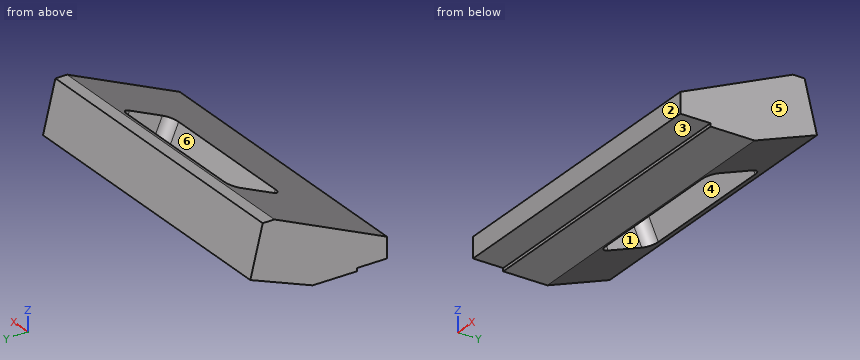
```python
from build123d import *

# Parameters (mm, degrees)
F1_DEPTH = 300
F3_DEPTH = 106


with BuildPart() as f1:
    # F0 (on Right) → F1 (new body)
    with BuildSketch(Plane.YZ):
        Polygon((0, 0), (0, -20), (29.5, -20), (29.5, -23), (72.5, -23), (133.294737, 0), (121.198642, 48.514786), (109.755708, 48.514786), align=None)
    extrude(amount=F1_DEPTH)

    # F2 (on face) → F3 (cut)
    with BuildSketch(Plane(origin=(0, 0, 0), x_dir=(1, 0, 0), z_dir=(0, -0.40429, 0.914631))):
        with BuildLine():
            Line((220, 115), (80, 115))
            ThreePointArc((80, 115), (72.928932, 112.071068), (70, 105))
            Line((70, 105), (70, 70))
            ThreePointArc((70, 70), (72.928932, 62.928932), (80, 60))
            Line((80, 60), (220, 60))
            ThreePointArc((220, 60), (227.071068, 62.928932), (230, 70))
            Line((230, 70), (230, 105))
            ThreePointArc((230, 105), (227.071068, 112.071068), (220, 115))
        make_face()
    extrude(amount=-F3_DEPTH, mode=Mode.SUBTRACT)


solid = f1.part
```
For this review, take the finished solid that the model builds, in its own axes (mm). Face numbers are marked on the shaded views. A direction names the side the tool comes from. Coordinates: 2 decimals unless noted, no trailing zeros. Write each loop counter-clockwise with the first axis right and the second up, starting at its lowest first coordinate (ties: lowest second). Pieces come first, ordered by that corner, then holes. Notation, with made-up numbers: (42.25, -23) - (69.25, -23) arc R14 cw to (69.25, -10) - close; hole circle Ø1 at (32, 80). An arc over 180 degrees is marked (long way). Answer in a Markdown table with one row per item. Add a question column.
Q1. For P1, Ø1.5, axis at x = 186.5, z = -13, coming from the +Y side; P2, Ø5, axis at x = 164, y = 50.5, coming from the +Z side; P3, Ø3, axis at x = 43, z = 38.5, coming from the -Y side, all flat-tipped, find the tip position at first contact; note any pin that passes through.
Q2. For probe 1 along X at (y, z) = (90, 32); probe 2 along X at (y, z) = (113.5, 12); probe 3 along Y at (x, z) = (156, 22), list the stretches that pass through material, from the lowest coordinate up.
Q3. We need section C-C, the plane x = 184. State the section outline as (y, z) points.
Q4. Draft analysis for pull direction Y (two halves, no side actions). For the marked faces 1, 2 and 3, state which applies: +Y half, -Y half, draft (parallel to the pull), parting line (faces both ways), or undercut.
Q5. Tool access review of the marked faces 4, 5 and 6: name each direction out of +Z, -Z, +X, -X, +Y, -Y from which nothing blocks a thin tool from reaching the whole face with its end or side.
Q6. We need section A-A, the plane x = 62.5. State the section outline as (y, z) points.
Q7. We need section B-B, the plane y = 89. State the section outline as (x, z) points, and give its area (3 significant figures).
Answer list:
| question | item | result |
|---|---|---|
| 1 | P1 | stops at y = 71.68 |
| 1 | P2 | stops at z = 23.43 |
| 1 | P3 | stops at y = 83.71 |
| 2 | probe 1 | x = 0 to 70, 230 to 300 |
| 2 | probe 2 | x = 0 to 70.69, 229.31 to 300 |
| 2 | probe 3 | y = 49.77 to 55.88, 116.01 to 127.81 |
| 3 | outline | (0, -20) - (29.5, -20) - (29.5, -23) - (72.5, -23) - (75.3, -21.94) - (54.88, 24.26) - (0, 0) - close; (105.18, 46.49) - (126.82, -2.45) - (133.29, 0) - (121.2, 48.51) - (109.76, 48.51) - close |
| 4 | face 1 | undercut |
| 4 | face 2 | -Y half |
| 4 | face 3 | draft |
| 5 | face 4 | -Z |
| 5 | face 5 | +Z, -Z, +X, +Y, -Y |
| 5 | face 6 | +Z |
| 6 | outline | (0, -20) - (29.5, -20) - (29.5, -23) - (72.5, -23) - (133.29, 0) - (121.2, 48.51) - (109.76, 48.51) - (0, 0) - close |
| 7 | outline | (0, -16.76) - (70, -16.76) - (70, 39.34) - (0, 39.34) - close; (230, -16.76) - (300, -16.76) - (300, 39.34) - (230, 39.34) - close |
| 7 | area | 7,850 mm2 |
